The model under review builds one solid part; all positions refer to its coordinate system, in mm. A direction names the side the tool comes from. Round coordinates to 2 decimals unless told otherwise and drop trailing zeros. Write each loop counter-clockwise with the first axis right and the second up, starting at its lowest first coordinate (ties: lowest second). Pieces come first, ordered by that corner, then holes.
Item 1: Clearance check with flat-ended pins moving along their axes: pin 1 Ø17 at (y, z) = (76.2, -177.8) entering from +X; pin 2 Ø20.5 at (x, y) = (8.5, 73.5) entering from +Z; pin 3 Ø7.5 at (x, z) = (7, -15.5) entering from +Y; pin 4 Ø23 at (x, y) = (-28.5, 31.5) entering from -Z. State where each tip first meets the part, or that it passes through.
Item 2: Add section C-C (z = -140). Give the boundary of the cut face in (x, y), plus the area to 3 significant figures.
Item 3: Add section B-B (z = 0). Give the boundary of the cut face in (x, y), plus the area to 3 significant figures.
Item 4: Add section A-A (y = 76.2). Give the boundary of the cut face in (x, z), plus the area to 3 significant figures.
Item 5: Add section D-D (z = -177.8). Give the boundary of the cut face in (x, y), plus the area to 3 significant figures.
Item 6: Draft analysis for pull direction Z (two halves, no side actions). For faces 1 (the face through (-114, 0, 25.4)), 2 (the face through (-114, 25.4, -15)), 3 (the face through (-114, 37, -203.2)), 4 (the face through (-114.478, 0.628, 14.274)), state which applies: +Z half, -Z half, draft (parallel to the pull), parting line (faces both ways), or undercut.
Item 7: To check wall thickness, follow L1, parallel to Y at x = -110.75, z = 0; L2, parallel to X at y = 36.5, z = -90; L3, parallel to Y at x = -104.5, z = -174. State the ranges of each line that lie inside material, in increasing order.
Item 8: Machinability: for faces 5 (the face through (-114.48, 88.25, -185.48)), 6 (the face through (13, 25.4, -15)), 7 (the face through (-101.6, 25, -142)), 8 (the face through (0, 0, -15)), which of the approach directions +Z, -Z, +X, -X, +Y, -Y give a long, thin tool a straight path to every point of the face, cutting with its end or side? Answer none if there is none.
```python
from build123d import *

# Parameters (mm, degrees)
SKETCH1_W           = 82.55
SKETCH1_H           = 76.2
SKETCH1_R           = 14.2875
SKETCH1_W_2         = 25.4
SKETCH1_R_2         = 12.7
BOSS_EXTRUDE1_DEPTH = 25.4
SKETCH1_3_W         = 25.4
SKETCH1_3_H         = 76.2
BOSS_EXTRUDE2_DEPTH = 101.6
BOSS_EXTRUDE4_START = -127
SKETCH1_4_W         = 25.4
SKETCH1_4_H         = 76.2
SKETCH1_4_R         = 12.7
SKETCH1_4_R_2       = 14.2875
SKETCH1_4_W_2       = 82.55
BOSS_EXTRUDE4_DEPTH = 25.4
SKETCH2_W           = 82.55
SKETCH2_H           = 25.4
CUT_EXTRUDE1_DEPTH  = 274.566372202


with BuildPart() as part:
    # Sketch1 → Boss-Extrude1 (new body)
    # profile 1 of 3: a face of its own
    with BuildSketch(Plane(origin=(0, 0, 0), x_dir=(0, 0, -1), z_dir=(1, 0, 0))):
        with Locations((15.875, 12.7)):
            Rectangle(SKETCH1_W, SKETCH1_H)
        Circle(SKETCH1_R, mode=Mode.SUBTRACT)
    # profile 2 of 3: a face of its own
    with BuildSketch(Plane(origin=(0, 0, 0), x_dir=(0, 0, -1), z_dir=(1, 0, 0))):
        with Locations((69.85, 12.7)):
            Rectangle(SKETCH1_W_2, SKETCH1_H)
    # profile 3 of 3: a face of its own
    with BuildSketch(Plane(origin=(0, 0, 0), x_dir=(0, 0, -1), z_dir=(1, 0, 0))):
        Polygon((82.55, 50.8), (82.55, -25.4), (203.2, -25.4), (203.2, 101.6), (152.4, 101.6), (152.4, 50.8), align=None)
        with Locations((177.8, 0)):
            Circle(SKETCH1_R_2, mode=Mode.SUBTRACT)
        with Locations((177.8, 76.2)):
            Circle(SKETCH1_R, mode=Mode.SUBTRACT)
    extrude(amount=BOSS_EXTRUDE1_DEPTH)

    # Sketch1<3> → Boss-Extrude2 (add)
    with BuildSketch(Plane(origin=(0, 0, 0), x_dir=(0, 0, -1), z_dir=(1, 0, 0))):
        with Locations((69.85, 12.7)):
            Rectangle(SKETCH1_3_W, SKETCH1_3_H)
    extrude(amount=-BOSS_EXTRUDE2_DEPTH)

    # Sketch1<4> → Boss-Extrude4 (add)
    # profile 1 of 3: a face of its own
    with BuildSketch(Plane(origin=(0, 0, 0), x_dir=(0, 0, -1), z_dir=(1, 0, 0)).offset(BOSS_EXTRUDE4_START)):
        with Locations((69.85, 12.7)):
            Rectangle(SKETCH1_4_W, SKETCH1_4_H)
    # profile 2 of 3: a face of its own
    with BuildSketch(Plane(origin=(0, 0, 0), x_dir=(0, 0, -1), z_dir=(1, 0, 0)).offset(BOSS_EXTRUDE4_START)):
        Polygon((82.55, 50.8), (82.55, -25.4), (203.2, -25.4), (203.2, 101.6), (152.4, 101.6), (152.4, 50.8), align=None)
        with Locations((177.8, 0)):
            Circle(SKETCH1_4_R, mode=Mode.SUBTRACT)
        with Locations((177.8, 76.2)):
            Circle(SKETCH1_4_R_2, mode=Mode.SUBTRACT)
    # profile 3 of 3: a face of its own
    with BuildSketch(Plane(origin=(0, 0, 0), x_dir=(0, 0, -1), z_dir=(1, 0, 0)).offset(BOSS_EXTRUDE4_START)):
        with Locations((15.875, 12.7)):
            Rectangle(SKETCH1_4_W_2, SKETCH1_4_H)
        Circle(SKETCH1_4_R_2, mode=Mode.SUBTRACT)
    extrude(amount=BOSS_EXTRUDE4_DEPTH)

    # Sketch2 → Cut-Extrude1 (cut, through all)
    with BuildSketch(Plane(origin=(25.4, 0, 0), x_dir=(0, 0, -1), z_dir=(1, 0, 0))):
        with Locations((15.875, 38.1)):
            Rectangle(SKETCH2_W, SKETCH2_H)
    extrude(amount=-CUT_EXTRUDE1_DEPTH, mode=Mode.SUBTRACT)


solid = part.part
```
Numbers:
1. pin 1: passes through
1. pin 2: stops at z = -152.4
1. pin 3: stops at y = 25.4
1. pin 4: stops at z = -82.55
2. outline: (-127, -25.4) - (-101.6, -25.4) - (-101.6, 50.8) - (-127, 50.8) - close; (0, -25.4) - (25.4, -25.4) - (25.4, 50.8) - (0, 50.8) - close
2. area: 3,870 mm2
3. outline: (-127, -25.4) - (-101.6, -25.4) - (-101.6, -14.29) - (-127, -14.29) - close; (-127, 14.29) - (-101.6, 14.29) - (-101.6, 25.4) - (-127, 25.4) - close; (0, -25.4) - (25.4, -25.4) - (25.4, -14.29) - (0, -14.29) - close; (0, 14.29) - (25.4, 14.29) - (25.4, 25.4) - (0, 25.4) - close
3. area: 1,130 mm2
4. outline: (-127, -203.2) - (-101.6, -203.2) - (-101.6, -192.09) - (-127, -192.09) - close; (-127, -163.51) - (-101.6, -163.51) - (-101.6, -152.4) - (-127, -152.4) - close; (0, -203.2) - (25.4, -203.2) - (25.4, -192.09) - (0, -192.09) - close; (0, -163.51) - (25.4, -163.51) - (25.4, -152.4) - (0, -152.4) - close
4. area: 1,130 mm2
5. outline: (-127, -25.4) - (-101.6, -25.4) - (-101.6, -12.7) - (-127, -12.7) - close; (-127, 12.7) - (-101.6, 12.7) - (-101.6, 61.91) - (-127, 61.91) - close; (-127, 90.49) - (-101.6, 90.49) - (-101.6, 101.6) - (-127, 101.6) - close; (0, -25.4) - (25.4, -25.4) - (25.4, -12.7) - (0, -12.7) - close; (0, 12.7) - (25.4, 12.7) - (25.4, 61.91) - (0, 61.91) - close; (0, 90.49) - (25.4, 90.49) - (25.4, 101.6) - (0, 101.6) - close
5. area: 3,710 mm2
6. face 1: +Z half
6. face 2: draft
6. face 3: -Z half
6. face 4: undercut
7. L1: y = -25.4 to -14.29, 14.29 to 25.4
7. L2: x = -127 to -101.6, 0 to 25.4
7. L3: y = -25.4 to -12.12, 12.12 to 62.43, 89.97 to 101.6
8. face 5: +X, -X
8. face 6: +Z, +X, -X, +Y
8. face 7: -Z, +Y, -Y
8. face 8: +Z, +Y, -Y
